The listing builds one solid part. Answer for the finished solid, in the listing's coordinates (mm). A direction names the side the tool comes from. Coordinates: 2 decimals unless noted, no trailing zeros. Order: outer loops, then holes, each group sorted by start corner. A loop starts at its lowest first (then second) coordinate and runs counter-clockwise, first axis right, second up. Notation, with made-up numbers: (76, 72) -> (92, 72) arc R32 cw to (92, 106) -> close; hole circle Ø7 at (8, 15.25). An arc over 180 degrees is marked (long way). Return JSON: item names as keys, results as strings.
Autodesk Inventor part; units mm, degrees
ref_plane "Work Plane1" through (0, 0, -15.5) normal (0, 0, 1) x (1, 0, 0)
ref_plane "YZ Plane" through (0, 0, 0) normal (1, 0, 0) x (0, 1, 0)
ref_plane "XZ Plane" through (0, 0, 0) normal (0, 1, 0) x (-1, 0, 0)
ref_plane "Work Plane1" through (0, 0, -15.5) normal (0, 0, 1) x (1, 0, 0)
sketch "Sketch1" plane through (0, 0, -15.5) normal (0, 0, 1) x (1, 0, 0)
  arc A0 (3.2082, 10) -> (16.2082, 10) centre (9.7082, 10) ccw
  line L0 (16.2082, 24) -> (16.2082, 10)
  line L1 (3.2082, 10) -> (3.2082, 24)
  arc A1 (16.2082, 24) -> (3.2082, 24) centre (9.7082, 24) ccw
extrude "Extrusion3" add sketch "Sketch1" along normal blind 1.5
sketch "Sketch2" plane through (0, 0, -14) normal (0, 0, 1) x (1, 0, 0)
  circle A0 centre (9.7082, 10) radius 2.5
extrude "Extrusion2" add sketch "Sketch2" along normal blind 1
sketch "Sketch3" plane through (0, 0, -14) normal (0, 0, 1) x (1, 0, 0)
  circle A0 centre (9.7082, 24) radius 2.5
extrude "Extrusion1" add sketch "Sketch3" along normal blind 1
hole "Hole2" at (9.7082, 10, -15.5) direction (0, 0, 1) diameter 3 depth 2.5
sketch "Sketch4" plane through (0, 0, -15.5) normal (0, 0, 1) x (1, 0, 0)
  point P0 (9.7082, 10)
hole "Hole1" at (9.7082, 24, -15.5) direction (0, 0, 1) diameter 3 depth 2.5
sketch "Sketch5" plane through (0, 0, -15.5) normal (0, 0, 1) x (1, 0, 0)
  point P0 (9.7082, 24)
1. Each of these flat-tipped pins is pushed along its axis until it touches: pin 1 Ø1.5 at (x, z) = (5, -14.5) entering from -Y; pin 2 Ø3 at (x, y) = (8.5, 16.5) entering from +Z; pin 3 Ø2.5 at (x, y) = (9.71, 10) entering from -Z. Where does it stop, or does it pass through?
Answer block:
{"pin 1": "stops at y = 4.84", "pin 2": "stops at z = -14", "pin 3": "passes through"}
2. The part is cut by section C-C on z = -13.7. Give the vertices of the cut face in (x, y).
Answer block:
{"outline": "circle Ø5 at (9.71, 10); circle Ø5 at (9.71, 24); hole circle Ø3 at (9.71, 10); hole circle Ø3 at (9.71, 24)"}
3. The part is cut by section A-A on x = 10.25. Give the vertices of the cut face in (y, z).
Answer block:
{"outline": "(3.52, -15.5) -> (8.6, -15.5) -> (8.6, -13) -> (7.56, -13) -> (7.56, -14) -> (3.52, -14) -> close; (11.4, -15.5) -> (22.6, -15.5) -> (22.6, -13) -> (21.56, -13) -> (21.56, -14) -> (12.44, -14) -> (12.44, -13) -> (11.4, -13) -> close; (25.4, -15.5) -> (30.48, -15.5) -> (30.48, -14) -> (26.44, -14) -> (26.44, -13) -> (25.4, -13) -> close"}
4. The part is cut by section B-B on y = 24.75. Give the vertices of the cut face in (x, z), and give its area (3 significant figures).
Answer block:
{"outline": "(3.25, -15.5) -> (8.41, -15.5) -> (8.41, -13) -> (7.32, -13) -> (7.32, -14) -> (3.25, -14) -> close; (11.01, -15.5) -> (16.16, -15.5) -> (16.16, -14) -> (12.09, -14) -> (12.09, -13) -> (11.01, -13) -> close", "area": "17.6 mm2"}
5. For faces 1 (the face through (10, 17, -15.5)), 2 (the face through (11.05, 21.89, -13.51)), determine the directions among +Z, -Z, +X, -X, +Y, -Y from which every point of the face is accessible in a straight line to the end or side of a thin tool.
Answer block:
{"face 1": "-Z, +X, -X, +Y, -Y", "face 2": "+Z"}
6. The part is cut by section D-D on x = 7.75. Give the vertices of the cut face in (y, z).
Answer block:
{"outline": "(3.8, -15.5) -> (30.2, -15.5) -> (30.2, -14) -> (25.55, -14) -> (25.55, -13) -> (22.45, -13) -> (22.45, -14) -> (11.55, -14) -> (11.55, -13) -> (8.45, -13) -> (8.45, -14) -> (3.8, -14) -> close"}
7. Consider line 1 (X direction, y = 10, z = -14.4); line 2 (Z direction, x = 14, y = 19); line 3 (X direction, y = 23.5, z = -14.8). Determine where each line is inside the solid, lowest interval first. Write a range as from..to.
Answer block:
{"line 1": "x = 3.21..8.21, 11.21..16.21", "line 2": "z = -15.5..-14", "line 3": "x = 3.21..8.29, 11.12..16.21"}
8. Determine the mould class of faces 3 (the face through (9.64, 22.5, -14.23)), 4 (the face through (16.208, 17, -15)), 5 (the face through (10.86, 12.22, -13.51)) for opening direction X: pulls with the +X half, pulls with the -X half, needs draft (parallel to the pull), parting line crosses it, or undercut.
Answer block:
{"face 3": "undercut", "face 4": "pulls with the +X half", "face 5": "parting line crosses it"}
